```python
from build123d import *


with BuildPart() as part:
    # Sketch1 → Revolve1 (revolve)
    with BuildSketch(Plane.XY, mode=Mode.PRIVATE) as revolve1_sk:
        with BuildLine():
            ThreePointArc((10, 35), (11.464466094, 31.464466094), (15, 30))
            Line((15, 30), (20, 30))
            ThreePointArc((20, 30), (23.535533906, 28.535533906), (25, 25))
            Line((25, 25), (34, 25))
            Line((34, 25), (35, 24))
            Line((35, 24), (35, 20))
            Line((35, 20), (50, 20))
            ThreePointArc((50, 20), (51.464466094, 16.464466094), (55, 15))
            Line((55, 15), (62.25, 15))
            Line((62.25, 15), (69.5, 7.5))
            ThreePointArc((69.5, 7.5), (74.803300859, 5.303300859), (77, 0))
            Line((77, 0), (0, 0))
            Line((0, 0), (0, 42.5))
            Line((0, 42.5), (9, 42.5))
            Line((9, 42.5), (10, 41.5))
            Line((10, 41.5), (10, 35))
        make_face()
    revolve(revolve1_sk.sketch.rotate(Axis((0, 0, 0), (1, 0, 0)), 90), axis=Axis((0, 0, 0), (1, 0, 0)))


solid = part.part
```
Can you work these out from the model? Positions are in its coordinate system, mm. A direction names the side the tool comes from. Coordinates: 2 decimals unless noted, no trailing zeros. Order: outer loops, then holes, each group sorted by start corner. A loop starts at its lowest first (then second) coordinate and runs counter-clockwise, first axis right, second up.
1. I need wall thicknesses on line 1 (X direction, y = -22, z = 30); line 2 (X direction, y = 10.5, z = -21.5); line 3 (Y direction, x = 3, z = 37.5). Which ranges of each line are inside material? Lowest first, please.
2. I'm going to push flat-ended pins straight in: pin 1 (12 mm diameter, centred on x = 37.5, z = 25, fed in from +Y); pin 2 (1 mm diameter, centred on x = 18.5, z = -25, fed in from -Y); pin 3 (8 mm diameter, centred on y = -8, z = 3.5, fed in from +X). Where does each tip first touch, or does it pass through?
3. If we section it at A-A (y = 0): Please give me the cut outline in (x, z).
4. For faces 1 (the face through (0, -1, 1)), 2 (the face through (58.68, -12.65, 8.06)), which set-ups out of +Z, -Z, +X, -X, +Y, -Y let a thin tool reach every point of the face, with its end or its side?
5. If we section it at D-D (x = 53): Please give me the cut outline in (y, z).
6. If we section it at C-C (x = 22): Please give me the cut outline in (y, z).
Entries:
1. line 1: x = 0 to 10
1. line 2: x = 0 to 35
1. line 3: y = -20 to 20
2. pin 1: stops at y = 14.83
2. pin 2: stops at y = -17.31
2. pin 3: stops at x = 75.32
3. outline: (0, -42.5) - (9, -42.5) - (10, -41.5) - (10, -35) arc R5 cw to (15, -30) - (20, -30) arc R5 ccw to (25, -25) - (34, -25) - (35, -24) - (35, -20) - (50, -20) arc R5 cw to (55, -15) - (62.25, -15) - (69.5, -7.5) arc R7.5 ccw to (69.5, 7.5) - (62.25, 15) - (55, 15) arc R5 cw to (50, 20) - (35, 20) - (35, 24) - (34, 25) - (25, 25) arc R5 ccw to (20, 30) - (15, 30) arc R5 cw to (10, 35) - (10, 41.5) - (9, 42.5) - (0, 42.5) - close
4. face 1: +Z, -Z, -X, +Y, -Y
4. face 2: +X
5. outline: circle Ø30.83 at (0, 0)
6. outline: circle Ø59.17 at (0, 0)
